Part model, mm, in its own coordinate system. Face numbers are marked on the shaded views. A direction names the side the tool comes from. Coordinates: 2 decimals unless noted, no trailing zeros. Loops run counter-clockwise (first coordinate to the right, second up) from the corner with the lowest first, then second, coordinate; pieces in that order, holes last. Notation, with made-up numbers: (78, -11.5) - (95, -11.5) arc R29 ccw to (95, 24.5) - close; hole circle Ø11 at (40, 73.5). An arc over 180 degrees is marked (long way). Answer as CSV lines item,"result".
Autodesk Inventor part; units mm, degrees
ref_plane "YZ Plane" through (0, 0, 0) normal (1, 0, 0) x (0, 1, 0)
ref_plane "XZ Plane" through (0, 0, 0) normal (0, 1, 0) x (-1, 0, 0)
ref_plane "XY Plane" through (0, 0, 0) normal (0, 0, 1) x (1, 0, 0)
sketch "Sketch1" plane through (0, 0, 0) normal (0, 1, 0) x (-1, 0, 0)
  point P0 (0, 0)
sketch "Sketch2" plane through (0, 0, 0) normal (1, 0, 0) x (0, 1, 0)
  line L0 (0, 0) -> (0, -65)
  line L1 (0, -65) -> (10, -65)
  line L2 (10, -65) -> (0, 0)
  dimension "d0" = 65
  dimension "d2" = 10
extrude "Extrusion1" add sketch "Sketch2" along normal blind 100
sketch "Sketch3" plane through (100, 0, 0) normal (1, 0, 0) x (0, 0, -1)
  line L0 (65, 10) -> (0, 0)
  line L1 (0, 0) -> (24, 0)
  line L2 (24, 0) -> (24, 3.6923)
  line L3 (24, 10) -> (0, 10)
  line L4 (0, 10) -> (0, 0)
  circle A0 centre (4, 4) radius 2.15
  circle A1 centre (12, 4) radius 2.15
  circle A2 centre (20, 4) radius 2.15
  line L5 (24, 10) -> (65, 10)
  line L6 (24, 3.6923) -> (65, 10)
  point P0 (0, 5)
  point P1 (12, 0)
  dimension "d5" = 24
  dimension "d6" = 10
  dimension "d7" = 4.3
  dimension "d9" = 4
  dimension "d10" = 4.3
  dimension "d11" = 8
  dimension "d12" = 4.3
  dimension "d13" = 8
  dimension "d38" = 4
  dimension "d39" = 4
  dimension "d40" = 4
sketch "Sketch4" plane through (0, 0, -65) normal (0, -1, 0) x (1, 0, 0)
  line L0 (0, 65) -> (100, 65)
  line L1 (85, 65) -> (90, 65)
  line L2 (100, 65) -> (100, 0)
  line L3 (85, 65) -> (100, 65)
  line L4 (100, 65) -> (100, 41)
  line L5 (100, 41) -> (90, 41)
  line L6 (100, 41) -> (90, 41)
  line L7 (90, 41) -> (90, 65)
  line L8 (90, 65) -> (100, 65)
  line L9 (100, 65) -> (100, 41)
  dimension "d24" = 10
extrude "Extrusion2" cut sketch "Sketch4" against normal blind 5
extrude "Extrusion3" add sketch "Sketch3" against normal blind 5 contours L0 A2 A1 L4 L3 L5 | L2 L1 L0 A1 A2
sketch "Sketch5" plane through (0, 0, -65) normal (0, -1, 0) x (1, 0, 0)
  line L0 (0, 65) -> (10, 65)
  line L1 (10, 65) -> (10, 41)
  line L2 (10, 41) -> (0, 41)
  line L3 (0, 41) -> (0, 65)
  dimension "d25" = 10
  dimension "d26" = 24
extrude "Extrusion4" cut sketch "Sketch5" against normal blind 5
sketch "Sketch6" plane through (0, 0, 0) normal (-1, 0, 0) x (0, 0, 1)
  line L0 (-65, 0) -> (-65, 10)
  line L1 (0, 0) -> (-65, 0)
  line L2 (-65, 0) -> (-65, 10)
  line L3 (-65, 10) -> (0, 10)
  line L4 (0, 10) -> (0, 0)
  circle A0 centre (-4, 4) radius 2.15
  circle A1 centre (-12, 4) radius 2.15
  circle A2 centre (-20, 4) radius 2.15
  dimension "d29" = 4.3
  dimension "d30" = 4
  dimension "d31" = 4
  dimension "d32" = 4.3
  dimension "d33" = 8
  dimension "d34" = 4.3
  dimension "d35" = 8
extrude "Extrusion5" add sketch "Sketch6" against normal blind 5
sketch "Sketch7" plane through (10, 0, -24) normal (0, 0, 1) x (1, 0, 0)
  line L0 (-5, 10) -> (85, 10)
  line L1 (0, 0) -> (0, 3.6923)
  line L2 (-5, 10) -> (0, 3.6923)
  line L3 (-5, 3.6923) -> (0, 3.6923)
  line L4 (0, 3.6923) -> (-5, 3.6923)
  line L5 (-5, 3.6923) -> (-5, 10)
  point P0 (-10, 0)
extrude "Extrusion6" add sketch "Sketch7" against normal blind 41
sketch "Sketch8" plane through (90, 0, -24) normal (0, 0, 1) x (1, 0, 0)
  line L0 (0, 3.6923) -> (5, 3.6923)
  line L1 (5, 3.6923) -> (5, 10)
  line L2 (0, 3.6923) -> (5, 10)
  line L3 (5, 10) -> (5, 3.6923)
  line L4 (5, 3.6923) -> (0, 3.6923)
  point P0 (-90, 0)
extrude "Extrusion7" add sketch "Sketch8" against normal blind 41
properties part number "slope"
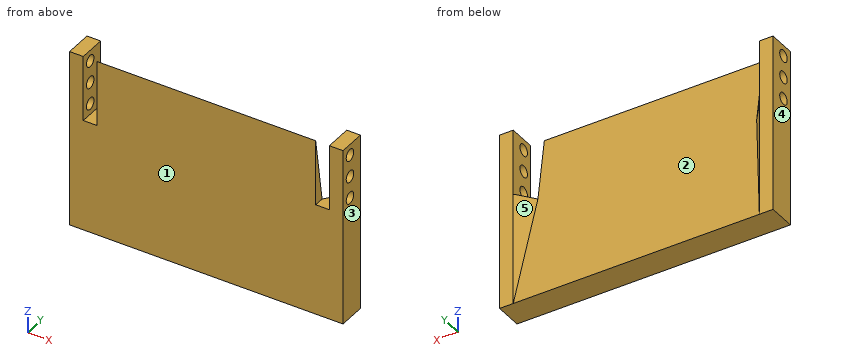
Q1. Saw through at A-A (z = -5). Give the cut face in (x, y), then the cut area to 3 significant figures.
Results:
outline,"(0, 0) - (5, 0) - (5, 2.1) - (0, 2.1) - close; (0, 5.9) - (5, 5.9) - (5, 10) - (0, 10) - close; (10, 0) - (90, 0) - (90, 0.77) - (10, 0.77) - close; (95, 0) - (100, 0) - (100, 2.1) - (95, 2.1) - close; (95, 5.9) - (100, 5.9) - (100, 10) - (95, 10) - close"
area,"123 mm^2"
Q2. Which spindle directions (+Z, -Z, +X, -X, +Y, -Y) get a long thin tool onto all of the face, cutting with end or side? Do the marked faces 1 and 2. Say none if no direction does.
Results:
face 1,"+Z, -Z, +X, -X, -Y"
face 2,"+Z, +Y"
Q3. Saw through at B-B (z = -12). Give the cut face in (x, y), then the cut area to 3 significant figures.
Results:
outline,"(0, 0) - (5, 0) - (5, 1.85) - (0, 1.85) - close; (0, 6.15) - (5, 6.15) - (5, 10) - (0, 10) - close; (10, 0) - (90, 0) - (90, 1.85) - (10, 1.85) - close; (95, 0) - (100, 0) - (100, 1.85) - (95, 1.85) - close; (95, 6.15) - (100, 6.15) - (100, 10) - (95, 10) - close"
area,"205 mm^2"
Q4. Wall check: L1, parallel to X at y = 1, z = -17; L2, parallel to X at y = 9.25, z = -2.5; L3, parallel to Y at x = 2.25, z = -20. Give the ranges that are in metal, low to high.
Results:
L1,"x = 0 to 5, 10 to 90, 95 to 100"
L2,"x = 0 to 5, 95 to 100"
L3,"y = 0 to 1.85, 6.15 to 10"
Q5. Saw through at D-D (x = 9). Give the cut face in (y, z).
Results:
outline,"(0, -65) - (10, -65) - (4.95, -32.2) - (4.95, -24) - (0, -24) - close"
Q6. Saw through at C-C (y = 8.25). Give the cut face in (x, z) (3 decimals).
Results:
outline,"(0, -65) - (100, -65) - (100, 0) - (95, 0) - (95, -24) - (93.613, -24) - (93.613, -53.625) - (6.387, -53.625) - (6.387, -24) - (5, -24) - (5, 0) - (0, 0) - close"
Q7. Flat gauge pins, fed straight in: pin 1 (4 mm diameter, centred on y = 4, z = -20, fed in from -X); pin 2 (4 mm diameter, centred on y = 4, z = -20, fed in from +X). Where does each tip first touch, or does it go through?
Results:
pin 1,"stops at x = 10"
pin 2,"stops at x = 90"
Q8. Two-plate mould, pull along X, no slides. Class the marked faces 3, 4 and 5: released by +X, released by -X, zero draft, split by the parting line, or undercut.
Results:
face 3,"released by +X"
face 4,"released by -X"
face 5,"undercut"
